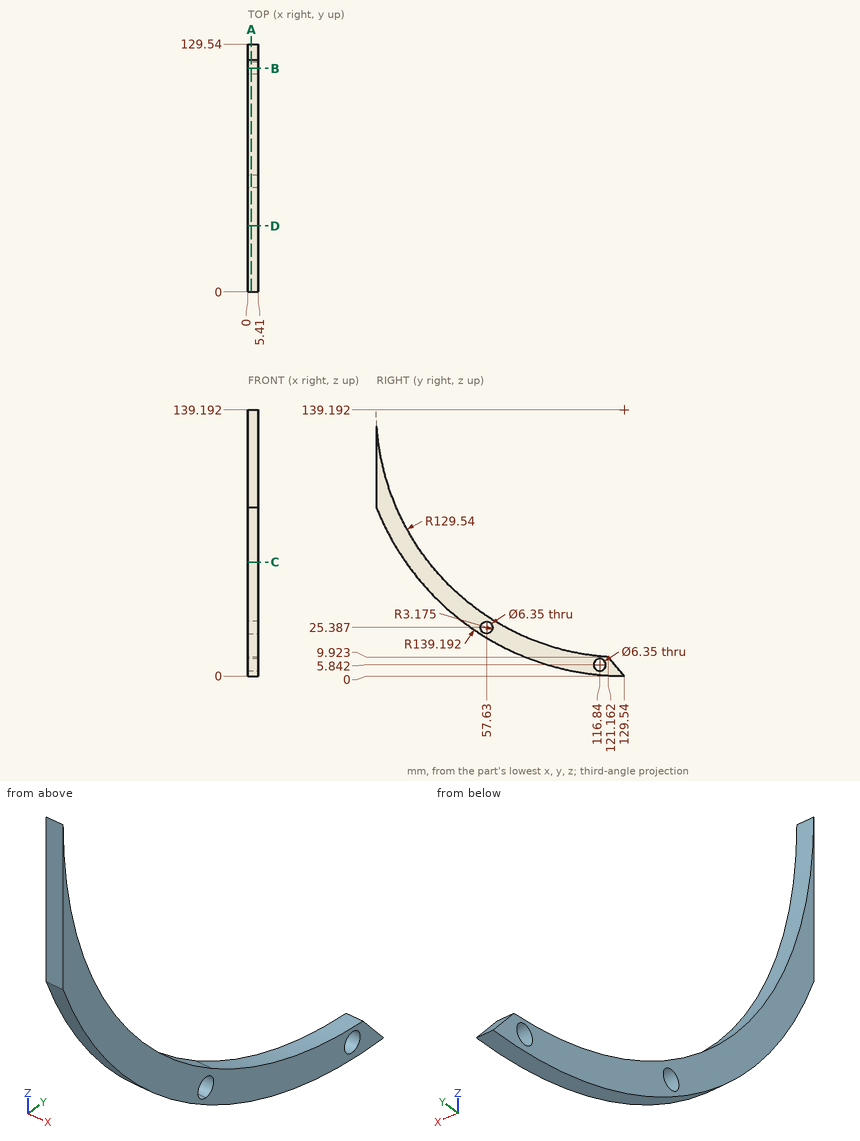
Answer from the drawing. Dimensions are ordinates in mm from the lowest x, y and z of the part. Round coordinates to 2 decimals unless told otherwise and drop trailing zeros. Order: outer loops, then holes, each group sorted by start corner. A loop starts at its lowest first (then second) coordinate and runs counter-clockwise, first axis right, second up. Notation, with made-up numbers: (50.25, -6.5) - (59.25, -6.5) arc R36 cw to (59.25, 29.5) - close; hole circle Ø5 at (70, -12). An arc over 180 degrees is marked (long way). Put each result on its own line as item: value. Start each with the question number.
(1) Find section A-A (x = 1.8). State how many separate pieces and enclosed holes the cut face has, plus the area to 3 significant figures.
(2) Straight lines are drawn through the part: probe 1 along Z at (x, y) = (3.75, 19) (1 decimal); probe 2 along Y at (x, z) = (0.9, 132); probe 3 along Z at (x, y) = (2.2, 108.5). For each, find the intervals that lie inside material, in ascending order. Write a range as from..to.
(3) Find section B-B (y = 116.84). Give the vertices of the cut face in (x, z), plus the area to 3 significant figures.
(4) Find section D-D (y = 34.5). Give the vertices of the cut face in (x, z).
(5) Find section C-C (z = 59.5). Give the vertices of the cut face in (x, y).
(6) Given P1, Ø5, axis at y = 27, z = 68, coming from the -X side; P2, Ø3, axis at x = 3, y = 100.5, coming from the +Z side; P3, Ø1.5, axis at x = 4, y = 77, coming from the +Z side, each flat-ended and moving along its own axis, determine where each tip first touches the part or whether it passes through.
Reply:
1. separate pieces: 1
1. enclosed holes: 2
1. area: 1,600 mm^2
2. probe 1: 54.6..71.7
2. probe 2: 0..0.2
2. probe 3: 1.6..11.37
3. outline: (0, 0.58) - (5.41, 0.58) - (5.41, 2.67) - (0, 2.67) - close; (0, 9.02) - (5.41, 9.02) - (5.41, 10.28) - (0, 10.28) - close
3. area: 18.1 mm^2
4. outline: (0, 37.5) - (5.41, 37.5) - (5.41, 51.17) - (0, 51.17) - close
5. outline: (0, 15.42) - (5.41, 15.42) - (5.41, 27.41) - (0, 27.41) - close
6. P1: through
6. P2: z = 13.3
6. P3: z = 21.12
